The model under review builds one solid part; all positions refer to its coordinate system, in mm. A direction names the side the tool comes from. Coordinates: 2 decimals unless noted, no trailing zeros. Order: outer loops, then holes, each group sorted by start corner. A loop starts at its lowest first (then second) coordinate and runs counter-clockwise, first axis right, second up.
```python
from build123d import *

# Parameters (mm, degrees)
F1_W     = 5
F1_H     = 6
F2_DEPTH = 10
F1_W_2   = 25
F3_START = 3
F1_W_3   = 43
F3_DEPTH = 7
F5_D     = 4.25
F5_DEPTH = 4
F5_TIP   = 1.2768288154
F6_D     = 4.25
F6_DEPTH = 4
F6_TIP   = 1.2768288154
F7_R     = 1.5
F8_R     = 0.5


with BuildPart() as f2:
    # F1 (on Top) → F2 (new body)
    with BuildSketch(Plane.XY):
        Polygon((36, 43), (26.5, 43), (26.5, 22), (26.5, 16), (36, 16), align=None)
        with Locations((24, 19)):
            Rectangle(F1_W, F1_H)
    extrude(amount=F2_DEPTH)



with BuildPart() as f2b:
    # F1 (on Top) → F2, piece 2 (new body)
    with BuildSketch(Plane.XY):
        Polygon((-46.5, 16), (-46.5, 22), (-46.5, 43), (-56, 43), (-56, 16), align=None)
        with Locations((-34, 19)):
            Rectangle(F1_W_2, F1_H)
    extrude(amount=F2_DEPTH)


with BuildPart() as f2_1:
    add(f2.part)

    add(f2b.part)  # F3 merges F2b
    # F1 (on Top) → F3 (join)
    with BuildSketch(Plane.XY.offset(F3_START)):
        with Locations((0, 19)):
            Rectangle(F1_W_3, F1_H)
    extrude(amount=F3_DEPTH)

    # F5
    with Locations(Plane(origin=(0, 43, 0), x_dir=(-1, 0, 0), z_dir=(0, 1, 0))):
        with Locations((-31.25, 4.25), (51.25, 4.25)):
            Hole(F5_D / 2, depth=F5_DEPTH)
            with Locations((0, 0, -(F5_DEPTH + F5_TIP / 2))):  # 118° drill point
                Cone(0, F5_D / 2, F5_TIP, mode=Mode.SUBTRACT)

    # F6
    with Locations(Plane(origin=(0, 0, 0), x_dir=(1, 0, 0), z_dir=(0, 0, -1))):
        with Locations((24.5, -19), (-24.5, -19)):
            Hole(F6_D / 2, depth=F6_DEPTH)
            with Locations((0, 0, -(F6_DEPTH + F6_TIP / 2))):  # 118° drill point
                Cone(0, F6_D / 2, F6_TIP, mode=Mode.SUBTRACT)

    # F7
    f7_edges = [f2_1.edges().sort_by_distance(p)[0] for p in [
        (26.5, 22, 5),
        (-46.5, 22, 5),
        (36, 16, 5),
        (-56, 16, 5),
        (21.5, 22, 1.5),
        (21.5, 16, 1.5),
        (-21.5, 22, 1.5),
        (-21.5, 16, 1.5),
    ]]
    fillet(f7_edges, radius=F7_R)

    # F8
    f8_edges = [f2_1.edges().sort_by_distance(p)[0] for p in [
        (36, 43, 5),
        (26.5, 43, 5),
        (-46.5, 43, 5),
        (-56, 43, 5),
    ]]
    fillet(f8_edges, radius=F8_R)


solid = f2_1.part
```
(1) Draft analysis for pull direction Z (two halves, no side actions). For faces 6 (the face through (33.213, 40.972, 3.436)), 7 (the face through (0, 19, 3)), 8 (the face through (31.619, 37.945, 4.266)), 9 (the face through (26.5, 33, 5)), state which applies: released by +Z, released by -Z, zero draft, split by the parting line, or undercut.
A:
face 6: undercut
face 7: released by -Z
face 8: undercut
face 9: zero draft
(2) We need section D-D, the plane x = 2.5. Write out the cut boundary in (y, z).
A:
outline: (16, 3) - (22, 3) - (22, 10) - (16, 10) - close
(3) Wall thickness on probe 1 along X at (y, z) = (40.55, 4.25) (3 decimals); probe 2 along X at (y, z) = (19, 0.95) (3 decimals); probe 3 along X at (y, z) = (36.75, 1.25): over which ranges is each line inside the solid? List them lowest first.
A:
probe 1: x = -56 to -53.375, -49.125 to -46.5, 26.5 to 29.125, 33.375 to 36
probe 2: x = -56 to -26.625, -22.375 to -21.5, 21.5 to 22.375, 26.625 to 36
probe 3: x = -56 to -46.5, 26.5 to 36
(4) We need section A-A, the plane z = 1.25. Write out the cut boundary in (x, y) (3 decimals), and give its area (3 significant figures).
A:
outline: (-56, 17.5) arc R1.5 ccw to (-54.5, 16) - (-23, 16) arc R1.5 ccw to (-21.5, 17.5) - (-21.5, 20.5) arc R1.5 ccw to (-23, 22) - (-45, 22) arc R1.5 cw to (-46.5, 23.5) - (-46.5, 42.5) arc R0.5 ccw to (-47, 43) - (-55.5, 43) arc R0.5 ccw to (-56, 42.5) - close; (21.5, 17.5) arc R1.5 ccw to (23, 16) - (34.5, 16) arc R1.5 ccw to (36, 17.5) - (36, 42.5) arc R0.5 ccw to (35.5, 43) - (27, 43) arc R0.5 ccw to (26.5, 42.5) - (26.5, 23.5) arc R1.5 cw to (25, 22) - (23, 22) arc R1.5 ccw to (21.5, 20.5) - close; hole circle Ø4.25 at (-24.5, 19); hole circle Ø4.25 at (24.5, 19)
area: 662 mm2
(5) For pin 1 Ø2.5 at (x, z) = (31.25, 4.25) entering from +Y; pin 2 Ø3 at (x, z) = (-10, 6.5) entering from +Y; pin 3 Ø3.5 at (x, z) = (-51.25, 4.25) entering from +Y, all flat-tipped, find the tip position at first contact; note any pin that passes through.
A:
pin 1: stops at y = 38.47
pin 2: stops at y = 22
pin 3: stops at y = 38.77
(6) We need section B-B, the plane y = 34.5. Write out the cut boundary in (x, z), and give its area (3 significant figures).
A:
outline: (-56, 0) - (-46.5, 0) - (-46.5, 10) - (-56, 10) - close; (26.5, 0) - (36, 0) - (36, 10) - (26.5, 10) - close
area: 190 mm2
(7) Machinability: for faces 1 (the face through (-46.5, 33, 5)), 2 (the face through (-21.93, 21.55, 1.52)), 3 (the face through (-53.373, 40.972, 4.343)), 4 (the face through (-22.9, 17.6, 2)), 5 (the face through (21.95, 16.43, 1.52)), which of the approach directions +Z, -Z, +X, -X, +Y, -Y give a long, thin tool a straight path to every point of the face, cutting with its end or side? Answer none if there is none.
A:
face 1: +Z, -Z, +Y
face 2: -Z, +Y
face 3: +Y
face 4: -Z
face 5: -Z, -Y
(8) We need section C-C, the plane x = -39. Write out the cut boundary in (y, z).
A:
outline: (16, 0) - (22, 0) - (22, 10) - (16, 10) - close
